CAD build for the part. Positions are in the model's coordinates, mm. A direction names the side the tool comes from. Coordinates: 2 decimals unless noted, no trailing zeros. Order: outer loops, then holes, each group sorted by start corner. A loop starts at its lowest first (then second) coordinate and runs counter-clockwise, first axis right, second up. Notation, with made-up numbers: (56.5, -33.5) - (64.5, -33.5) arc R12 ccw to (64.5, -26.5) - close; hole circle Ø2 at (-26, 59). An arc over 180 degrees is marked (long way). Use one line per item in the form item = value.
```python
from build123d import *

# Parameters (mm, degrees)
SKETCH1_W                = 60.2
SKETCH1_H                = 160
BOSS_EXTRUDE1_DEPTH      = 6
SKETCH3_W                = 40
SKETCH3_H                = 5
BOSS_EXTRUDE2_DEPTH      = 15
BOSS_EXTRUDE3_DEPTH      = 5
BOSS_EXTRUDE3_DEPTH_BACK = 110
SKETCH4_R                = 18
SKETCH5_R                = 5
BOSS_EXTRUDE4_DEPTH      = 40
SKETCH6_R                = 8
BOSS_EXTRUDE5_DEPTH      = 36
CHAMFER1_SIZE            = 5
CHAMFER1_SIZE2           = 1.819851171
FILLET1_R                = 1.5


with BuildPart() as part:
    # Sketch1 → Boss-Extrude1 (new body)
    with BuildSketch(Plane(origin=(0, 0, 0), x_dir=(1, 0, 0), z_dir=(0, 1, 0))):
        with Locations((30.1, 80)):
            Rectangle(SKETCH1_W, SKETCH1_H)
        with BuildLine():
            Line((7.85, 152.55), (16.15, 152.55))
            ThreePointArc((16.15, 152.55), (19.6, 149.1), (16.15, 145.65))
            Line((16.15, 145.65), (7.85, 145.65))
            ThreePointArc((7.85, 145.65), (4.4, 149.1), (7.85, 152.55))
        make_face(mode=Mode.SUBTRACT)
        with BuildLine():
            Line((52.35, 145.65), (44.05, 145.65))
            ThreePointArc((44.05, 145.65), (40.6, 149.1), (44.05, 152.55))
            Line((44.05, 152.55), (52.35, 152.55))
            ThreePointArc((52.35, 152.55), (55.8, 149.1), (52.35, 145.65))
        make_face(mode=Mode.SUBTRACT)
        with BuildLine():
            Line((52.35, 7.45), (44.05, 7.45))
            ThreePointArc((44.05, 7.45), (40.6, 10.9), (44.05, 14.35))
            Line((44.05, 14.35), (52.35, 14.35))
            ThreePointArc((52.35, 14.35), (55.8, 10.9), (52.35, 7.45))
        make_face(mode=Mode.SUBTRACT)
        with BuildLine():
            Line((7.85, 14.35), (16.15, 14.35))
            ThreePointArc((16.15, 14.35), (19.6, 10.9), (16.15, 7.45))
            Line((16.15, 7.45), (7.85, 7.45))
            ThreePointArc((7.85, 7.45), (4.4, 10.9), (7.85, 14.35))
        make_face(mode=Mode.SUBTRACT)
    extrude(amount=BOSS_EXTRUDE1_DEPTH)

    # Sketch3 → Boss-Extrude2 (add)
    with BuildSketch(Plane(origin=(0, 6, 0), x_dir=(1, 0, 0), z_dir=(0, 1, 0))):
        with Locations((30.1, 130)):
            Rectangle(SKETCH3_W, SKETCH3_H)
        with Locations((30.1, 30)):
            Rectangle(SKETCH3_W, SKETCH3_H)
    extrude(amount=BOSS_EXTRUDE2_DEPTH)

    # Sketch4 → Boss-Extrude3 (add, two sides: drawn at the far end of the back side and taken through both)
    with BuildSketch(Plane(origin=(0, 0, -132.5), x_dir=(-1, 0, 0), z_dir=(0, 0, -1)).offset(-BOSS_EXTRUDE3_DEPTH_BACK)):
        with Locations((-30.1, 31)):
            Circle(SKETCH4_R)
    extrude(amount=BOSS_EXTRUDE3_DEPTH + BOSS_EXTRUDE3_DEPTH_BACK)

    # Sketch5 → Boss-Extrude4 (add)
    with BuildSketch(Plane.XY.offset(-22.5)):
        with Locations((30.1, 31)):
            Circle(SKETCH5_R)
    extrude(amount=BOSS_EXTRUDE4_DEPTH)

    # Sketch6 → Boss-Extrude5 (add)
    with BuildSketch(Plane.XY.offset(17.5)):
        with Locations((30.1, 31)):
            Circle(SKETCH6_R)
    extrude(amount=BOSS_EXTRUDE5_DEPTH)

    # Chamfer1
    chamfer1_edges = [part.edges().sort_by_distance(p)[0] for p in [
        (22.1, 31, 53.5),
    ]]
    chamfer1_side = [part.faces().sort_by_distance(p)[0] for p in [
        (22.1, 31, 35.5),
    ]]
    chamfer(chamfer1_edges, length=CHAMFER1_SIZE, length2=CHAMFER1_SIZE2, reference=chamfer1_side[0])

    # Fillet1
    fillet1_edges = [part.edges().sort_by_distance(p)[0] for p in [
        (25.1, 31, 17.5),
        (22.1, 31, 17.5),
    ]]
    fillet(fillet1_edges, radius=FILLET1_R - 0.0001)  # a hair under: the kernel refuses the full size


solid = part.part
```
Item 1: Two-plate mould, pull along X, no slides. Class faces 1 (the face through (30, 12, -127.5)), 2 (the face through (50.1, 13, -130)), 3 (the face through (12, 3, -145.65)): +X half, -X half, draft (parallel to the pull), parting line (faces both ways), or undercut.
Derived:
face_1 = draft
face_2 = +X half
face_3 = undercut
Item 2: Cut at C-C, the plane y = 10.5. Write the cut outline in (x, z), plus the area to 3 significant figures.
Derived:
outline = (10.1, -132.5) - (50.1, -132.5) - (50.1, -127.5) - (10.1, -127.5) - close; (10.1, -32.5) - (50.1, -32.5) - (50.1, -27.5) - (10.1, -27.5) - close
area = 400 mm²
Item 3: Cut at D-D, the plane z = -149.1. Write the cut outline in (x, y), plus the area to 3 significant figures.
Derived:
outline = (0, 0) - (4.4, 0) - (4.4, 6) - (0, 6) - close; (19.6, 0) - (40.6, 0) - (40.6, 6) - (19.6, 6) - close; (55.8, 0) - (60.2, 0) - (60.2, 6) - (55.8, 6) - close
area = 179 mm²
Item 4: Drill centre lines: line 1 (Z direction, x = 12, y = 6.5); line 2 (Y direction, x = 58.5, z = -75); line 3 (Y direction, x = 38, z = -73). Where is each one in solid material? Low to high. Write a range as [from, to].
Derived:
line_1 = [-132.5, -127.5], [-32.5, -27.5]
line_2 = [0, 6]
line_3 = [0, 6], [14.83, 47.17]
Item 5: Drop flat-ended pins along their axis: pin 1 (4 mm diameter, centred on x = 32, y = 31.5, fed in from -Z); pin 2 (5 mm diameter, centred on x = 47.5, y = 2, fed in from +Z); pin 3 (4 mm diameter, centred on y = 12.5, z = -129, fed in from -X); pin 4 (1.5 mm diameter, centred on x = 45, y = 43.5, fed in from -Z). Give the stop position or say it passes through.
Derived:
pin_1 = -137.5
pin_2 = 0
pin_3 = 10.1
pin_4 = through
Item 6: 3-axis set-ups, long thin cutter, end or side, ignore diameter. For faces 4 (the face through (48, 3, -145.65)), 5 (the face through (30, 31, -137.5)), 6 (the face through (30, 12, -132.5)): which of +Z, -Z, +X, -X, +Y, -Y reach the whole face in a straight line?
Derived:
face_4 = +Y, -Y
face_5 = -Z, +X, -X, +Y
face_6 = -Z
Item 7: Cut at B-B, the plane z = -10.9. Write the cut outline in (x, y), plus the area to 3 significant figures.
Derived:
outline = (0, 0) - (4.4, 0) - (4.4, 6) - (0, 6) - close; (19.6, 0) - (40.6, 0) - (40.6, 6) - (19.6, 6) - close; circle Ø10 at (30.1, 31); (55.8, 0) - (60.2, 0) - (60.2, 6) - (55.8, 6) - close
area = 257 mm²
